The listing builds one solid part. Answer for the finished solid, in the listing's coordinates (mm). Face numbers are marked on the shaded views. A direction names the side the tool comes from. Coordinates: 2 decimals unless noted, no trailing zeros. Write each loop counter-clockwise with the first axis right and the second up, starting at its lowest first coordinate (ties: lowest second). Pieces come first, ordered by that corner, then holes.
from build123d import *

# Parameters (mm, degrees)
CYLINDER001_R     = 2.1
CYLINDER001_DEPTH = 10
BOX002_W          = 9
BOX002_H          = 8
BOX002_DEPTH      = 10
BOX001_W          = 3
BOX001_H          = 12
BOX001_DEPTH      = 11
CYLINDER_R        = 2
CYLINDER_DEPTH    = 10
BOX_W             = 26
BOX_H             = 13
BOX_DEPTH         = 10
BOX_ROLL_ANGLE    = 90
CHAMFER_SIZE      = 1
CHAMFER001_SIZE   = 1
CHAMFER002_SIZE   = 1
CHAMFER003_SIZE   = 1
CHAMFER004_SIZE   = 1


with BuildPart() as cylinder001:
    # Cylinder001 → Cylinder001 (new body)
    with BuildSketch(Plane(origin=(5, -5, -5), x_dir=(1, 0, 0), z_dir=(0, 0, 1))):
        Circle(CYLINDER001_R)
    extrude(amount=CYLINDER001_DEPTH)


with BuildPart() as cube002:
    # Box002 → Box002 (new body)
    with BuildSketch(Plane(origin=(9, -9, -1), x_dir=(1, 0, 0), z_dir=(0, 0, 1))):
        with Locations((4.5, 4)):
            Rectangle(BOX002_W, BOX002_H)
    extrude(amount=BOX002_DEPTH)


with BuildPart() as cube001:
    # Box001 → Box001 (new body)
    with BuildSketch(Plane(origin=(20, -11, -1), x_dir=(1, 0, 0), z_dir=(0, 0, 1))):
        with Locations((1.5, 6)):
            Rectangle(BOX001_W, BOX001_H)
    extrude(amount=BOX001_DEPTH)


with BuildPart() as cylinder:
    # Cylinder → Cylinder (new body)
    with BuildSketch(Plane(origin=(5, -5, -5), x_dir=(1, 0, 0), z_dir=(0, 0, 1))):
        Circle(CYLINDER_R)
    extrude(amount=CYLINDER_DEPTH)


with BuildPart() as cut003:
    # Box → Box (new body)
    with BuildSketch(Plane.XY):
        with Locations((13, 6.5)):
            Rectangle(BOX_W, BOX_H)
    extrude(amount=BOX_DEPTH)


with BuildPart() as cut003_1:
    # Box roll: moved
    add(cut003.part.rotate(Axis((0, 0, 0), (1, 0, 0)), BOX_ROLL_ANGLE))


with BuildPart() as cut003_2:
    # Box placement: moved
    add(cut003_1.part)

    # Cut: cut Cylinder
    add(cylinder.part, mode=Mode.SUBTRACT)

    # Cut001: cut Cube001
    add(cube001.part, mode=Mode.SUBTRACT)

    # Chamfer
    chamfer_edges = [cut003_2.edges().sort_by_distance(p)[0] for p in [
        (0, -5, 0),
        (23, -5, 0),
    ]]
    chamfer(chamfer_edges, length=CHAMFER_SIZE)

    # Chamfer001
    chamfer001_edges = [cut003_2.edges().sort_by_distance(p)[0] for p in [
        (20, -5, 0),
    ]]
    chamfer(chamfer001_edges, length=CHAMFER001_SIZE)

    # Chamfer002
    chamfer002_edges = [cut003_2.edges().sort_by_distance(p)[0] for p in [
        (26, -5, 0),
    ]]
    chamfer(chamfer002_edges, length=CHAMFER002_SIZE)

    # Chamfer003
    chamfer003_edges = [cut003_2.edges().sort_by_distance(p)[0] for p in [
        (0, -5, 13),
    ]]
    chamfer(chamfer003_edges, length=CHAMFER003_SIZE)

    # Chamfer004
    chamfer004_edges = [cut003_2.edges().sort_by_distance(p)[0] for p in [
        (26, -5, 13),
    ]]
    chamfer(chamfer004_edges, length=CHAMFER004_SIZE)

    # Cut002: cut Cube002
    add(cube002.part, mode=Mode.SUBTRACT)

    # Cut003: cut Cylinder001
    add(cylinder001.part, mode=Mode.SUBTRACT)


solid = cut003_2.part
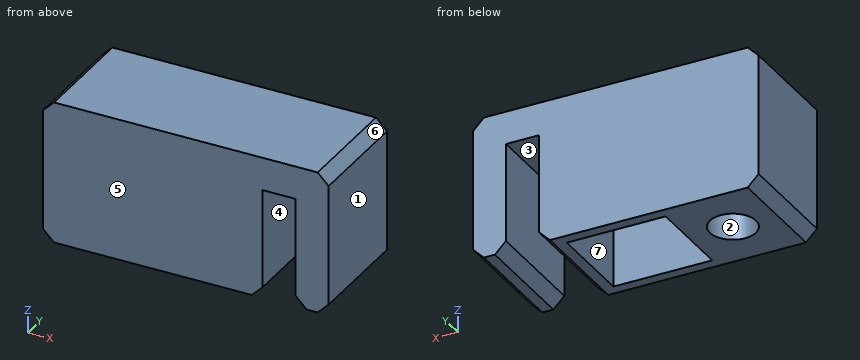
Q1. The part is cut by section B-B, the plane z = 5.5. Write down the section's boundary in (x, y), then the cut area to 3 significant figures.
Answers below:
outline: (0, -10) - (20, -10) - (20, 0) - (0, 0) - close; (23, -10) - (26, -10) - (26, 0) - (23, 0) - close; hole (9, -9) - (18, -9) - (18, -1) - (9, -1) - close
area: 158 mm2
Q2. Find the intervals of material crossed by probe 1 along X at (y, z) = (-5, 3.2); probe 2 along X at (y, z) = (-1.5, 8.25); probe 3 along Y at (x, z) = (5, 3.5), in increasing order.
Answers below:
probe 1: x = 0 to 2.9, 7.1 to 9, 18 to 20, 23 to 26
probe 2: x = 0 to 9, 18 to 20, 23 to 26
probe 3: y = -10 to -7.1, -2.9 to 0
Q3. The part is cut by section C-C, the plane y = -5. Write down the section's boundary in (x, z), then the cut area to 3 significant figures.
Answers below:
outline: (0, 1) - (1, 0) - (2.9, 0) - (2.9, 5) - (7.1, 5) - (7.1, 0) - (9, 0) - (9, 9) - (18, 9) - (18, 0) - (19, 0) - (20, 1) - (20, 10) - (23, 10) - (23, 1) - (24, 0) - (25, 0) - (26, 1) - (26, 12) - (25, 13) - (1, 13) - (0, 12) - close
area: 203 mm2
Q4. Determine the mould class of the marked faces 4, 5, 6 and 7 for opening direction X: released by +X, released by -X, zero draft, split by the parting line, or undercut.
Answers below:
face 4: undercut
face 5: zero draft
face 6: released by +X
face 7: undercut
Q5. The part is cut by section A-A, the plane z = 2. Write down the section's boundary in (x, y), then the cut area to 3 significant figures.
Answers below:
outline: (0, -10) - (20, -10) - (20, 0) - (0, 0) - close; (23, -10) - (26, -10) - (26, 0) - (23, 0) - close; hole circle Ø4.2 at (5, -5); hole (9, -9) - (18, -9) - (18, -1) - (9, -1) - close
area: 144 mm2
Q6. Which of the six approach directions +Z, -Z, +X, -X, +Y, -Y give full straight-line access (tool end or side, diameter ignored) to the marked faces 1, 2 and 3?
Answers below:
face 1: +Z, -Z, +X, +Y, -Y
face 2: -Z
face 3: -Z, +Y, -Y
Q7. Given pin 1 (2.5 mm diameter, centred on x = 13.5, y = -4.5, fed in from -Z); pin 2 (0.9 mm diameter, centred on x = 21.5, y = -6.5, fed in from -Z), each flat-ended and moving along its own axis, determine where each tip first touches the part or whether it passes through.
Answers below:
pin 1: stops at z = 9
pin 2: stops at z = 10
Q8. The part is cut by section D-D, the plane z = 9.25. Write down the section's boundary in (x, y), then the cut area to 3 significant figures.
Answers below:
outline: (0, -10) - (20, -10) - (20, 0) - (0, 0) - close; (23, -10) - (26, -10) - (26, 0) - (23, 0) - close
area: 230 mm2
